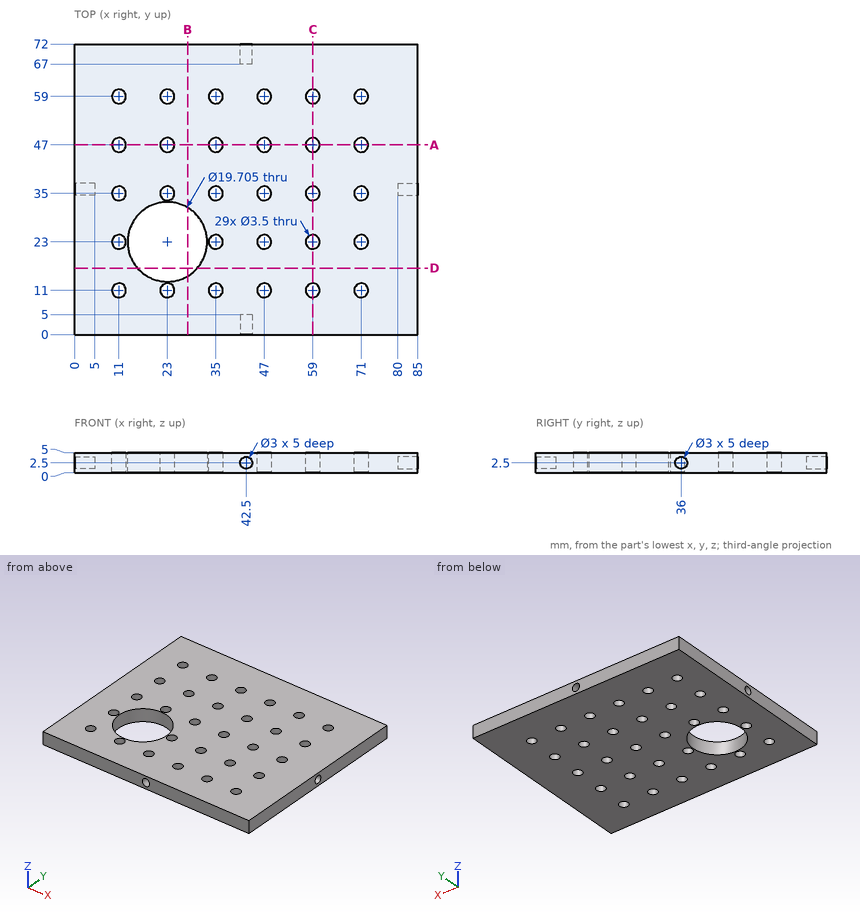
Could you check a few things on this drawing? It's one solid part, dimensions in mm from its lowest x, y, z. Round coordinates to 2 decimals unless told otherwise and drop trailing zeros. Write each loop counter-clockwise with the first axis right and the second up, starting at its lowest first coordinate (ties: lowest second). Pieces come first, ordered by that corner, then holes. Notation, with made-up numbers: M 46.25,16.25 L 86.25,16.25 A19 ccw 86.25,23.25 Z; hole C -28.75,59.5 d6. An arc over 180 degrees is marked long. Answer as CSV lines item,"result". Start each with the question number.
1. Suppose I cut it at B-B on x = 28. Write out the boundary of the cut face in (y, z), then the cut area to 3 significant figures.
2. Suppose I cut it at D-D on y = 16.5. Write out the boundary of the cut face in (x, z).
3. Suppose I cut it at A-A on y = 47. Write out the boundary of the cut face in (x, z), then the cut area to 3 significant figures.
4. Suppose I cut it at C-C on x = 59. Write out the boundary of the cut face in (y, z).
5. I'm going to push a flat-ended pin straight in: pin 1 Ø0.9 at (y, z) = (36, 2) entering from +X. Where does the tip first touch, or does it pass through?
6. I need wall thicknesses on probe 1 along Y at (x, z) = (59, 3.65); probe 2 along Y at (x, z) = (23, 1.1); probe 3 along Y at (x, z) = (17, 3.3) (1 decimal). Which ranges of each line are inside material? Lowest first, please.
Check result:
1,outline,"M 0,0 L 14.51,0 L 14.51,5 L 0,5 Z; M 31.49,0 L 72,0 L 72,5 L 31.49,5 Z"
1,area,"275 mm2"
2,outline,"M 0,0 L 15.6,0 L 15.6,5 L 0,5 Z; M 30.4,0 L 85,0 L 85,5 L 30.4,5 Z"
3,outline,"M 0,0 L 9.25,0 L 9.25,5 L 0,5 Z; M 12.75,0 L 21.25,0 L 21.25,5 L 12.75,5 Z; M 24.75,0 L 33.25,0 L 33.25,5 L 24.75,5 Z; M 36.75,0 L 45.25,0 L 45.25,5 L 36.75,5 Z; M 48.75,0 L 57.25,0 L 57.25,5 L 48.75,5 Z; M 60.75,0 L 69.25,0 L 69.25,5 L 60.75,5 Z; M 72.75,0 L 85,0 L 85,5 L 72.75,5 Z"
3,area,"320 mm2"
4,outline,"M 0,0 L 9.25,0 L 9.25,5 L 0,5 Z; M 12.75,0 L 21.25,0 L 21.25,5 L 12.75,5 Z; M 24.75,0 L 33.25,0 L 33.25,5 L 24.75,5 Z; M 36.75,0 L 45.25,0 L 45.25,5 L 36.75,5 Z; M 48.75,0 L 57.25,0 L 57.25,5 L 48.75,5 Z; M 60.75,0 L 72,0 L 72,5 L 60.75,5 Z"
5,pin 1,"stops at x = 80"
6,probe 1,"y = 0 to 9.25, 12.75 to 21.25, 24.75 to 33.25, 36.75 to 45.25, 48.75 to 57.25, 60.75 to 72"
6,probe 2,"y = 0 to 9.25, 12.75 to 13.15, 32.85 to 33.25, 36.75 to 45.25, 48.75 to 57.25, 60.75 to 72"
6,probe 3,"y = 0 to 15.2, 30.8 to 72"
